from build123d import *

# Parameters (mm, degrees)
SKETCH1_W           = 36.7
SKETCH1_H           = 34.9
SKETCH1_W_2         = 34.7
SKETCH1_H_2         = 32.9
BOSS_EXTRUDE1_DEPTH = 11.2
SKETCH2_W           = 4.9
SKETCH2_H           = 1
CUT_EXTRUDE1_DEPTH  = 1.9
SKETCH4_W           = 36.7
SKETCH4_H           = 34.9
BOSS_EXTRUDE3_DEPTH = 2.5
SKETCH5_W           = 14
SKETCH5_H           = 14
CUT_EXTRUDE2_DEPTH  = 14.7
SKETCH6_W           = 16
SKETCH6_H           = 16
SKETCH6_W_2         = 14
SKETCH6_H_2         = 14
BOSS_EXTRUDE4_DEPTH = 6


with BuildPart() as part:
    # Sketch1 → Boss-Extrude1 (new body)
    with BuildSketch(Plane.XY):
        with Locations((18.35, 17.45)):
            Rectangle(SKETCH1_W, SKETCH1_H)
        with Locations((18.35, 17.45)):
            Rectangle(SKETCH1_W_2, SKETCH1_H_2, mode=Mode.SUBTRACT)
    extrude(amount=BOSS_EXTRUDE1_DEPTH)

    # Sketch2 → Cut-Extrude1 (cut)
    with BuildSketch(Plane(origin=(0, 0, 0), x_dir=(-1, 0, 0), z_dir=(0, 0, -1))):
        with Locations((-28.25, 0.5)):
            Rectangle(SKETCH2_W, SKETCH2_H)
    extrude(amount=-CUT_EXTRUDE1_DEPTH, mode=Mode.SUBTRACT)

    # Sketch4 → Boss-Extrude3 (add)
    with BuildSketch(Plane.XY.offset(11.2)):
        with Locations((18.35, 17.45)):
            Rectangle(SKETCH4_W, SKETCH4_H)
    extrude(amount=BOSS_EXTRUDE3_DEPTH)

    # Sketch5 → Cut-Extrude2 (cut, through all)
    with BuildSketch(Plane.XY.offset(13.7)):
        with Locations((18.3, 18.3)):
            Rectangle(SKETCH5_W, SKETCH5_H)
    extrude(amount=-CUT_EXTRUDE2_DEPTH, mode=Mode.SUBTRACT)

    # Sketch6 → Boss-Extrude4 (add)
    with BuildSketch(Plane(origin=(0, 0, 11.2), x_dir=(-1, 0, 0), z_dir=(0, 0, -1))):
        with Locations((-18.3, 18.3)):
            Rectangle(SKETCH6_W, SKETCH6_H)
        with Locations((-18.3, 18.3)):
            Rectangle(SKETCH6_W_2, SKETCH6_H_2, mode=Mode.SUBTRACT)
    extrude(amount=BOSS_EXTRUDE4_DEPTH)


solid = part.part
Can you work these out from the model? Positions are in its coordinate system, mm. A direction names the side the tool comes from. Give positions to 0.01 mm unless a question says otherwise; leave off trailing zeros. Loops run counter-clockwise (first coordinate to the right, second up) from the corner with the lowest first, then second, coordinate; pieces in that order, holes last. Notation, with made-up numbers: (41, 66.25) -> (48, 66.25) arc R22 ccw to (48, 105.25) -> close; hole circle Ø7 at (-40, 6). An arc over 180 degrees is marked (long way). Use one line per item in the form item = value.
1) We'd pull the mould along Y, two halves only. Please class faces 1 (the face through (18, 34.9, 7)), 2 (the face through (30.7, 0.5, 0.9)), 3 (the face through (18, 1, 6)): released by +Y, released by -Y, zero draft, split by the parting line, or undercut.
Answers:
face_1 = released by +Y
face_2 = zero draft
face_3 = undercut
2) If we section it at D-D (z = 12.5): Please give me the cut outline in (x, y), plus the area to 3 significant figures.
Answers:
outline = (0, 0) -> (36.7, 0) -> (36.7, 34.9) -> (0, 34.9) -> close; hole (11.3, 11.3) -> (25.3, 11.3) -> (25.3, 25.3) -> (11.3, 25.3) -> close
area = 1,080 mm²
3) I need wall thicknesses on line 1 along Y through (x, z) = (15, 10.25); line 2 along Y through (x, z) = (4.5, 8.5); line 3 along X through (y, z) = (22, 13). Which ranges of each line are inside material? Lowest first, please.
Answers:
line_1 = 0 to 1, 10.3 to 11.3, 25.3 to 26.3, 33.9 to 34.9
line_2 = 0 to 1, 33.9 to 34.9
line_3 = 0 to 11.3, 25.3 to 36.7
4) If we section it at C-C (y = 12): Please give me the cut outline in (x, z).
Answers:
outline = (0, 0) -> (1, 0) -> (1, 11.2) -> (10.3, 11.2) -> (10.3, 5.2) -> (11.3, 5.2) -> (11.3, 13.7) -> (0, 13.7) -> close; (25.3, 5.2) -> (26.3, 5.2) -> (26.3, 11.2) -> (35.7, 11.2) -> (35.7, 0) -> (36.7, 0) -> (36.7, 13.7) -> (25.3, 13.7) -> close
5) If we section it at B-B (x = 22): Please give me the cut outline in (y, z).
Answers:
outline = (0, 0) -> (1, 0) -> (1, 11.2) -> (10.3, 11.2) -> (10.3, 5.2) -> (11.3, 5.2) -> (11.3, 13.7) -> (0, 13.7) -> close; (25.3, 5.2) -> (26.3, 5.2) -> (26.3, 11.2) -> (33.9, 11.2) -> (33.9, 0) -> (34.9, 0) -> (34.9, 13.7) -> (25.3, 13.7) -> close
6) If we section it at A-A (z = 8.75): Please give me the cut outline in (x, y), plus the area to 3 significant figures.
Answers:
outline = (0, 0) -> (36.7, 0) -> (36.7, 34.9) -> (0, 34.9) -> close; (10.3, 10.3) -> (26.3, 10.3) -> (26.3, 26.3) -> (10.3, 26.3) -> close; hole (1, 1) -> (35.7, 1) -> (35.7, 33.9) -> (1, 33.9) -> close; hole (11.3, 11.3) -> (25.3, 11.3) -> (25.3, 25.3) -> (11.3, 25.3) -> close
area = 199 mm²
7) Will these pins go through, and if not, where does the flat tip stop? pin 1 (0.8 mm diameter, centred on x = 28.5, y = 0.5, fed in from -Z); pin 2 (3.5 mm diameter, centred on y = 12, z = 6, fed in from -X); pin 3 (1.5 mm diameter, centred on x = 17.5, y = 6.5, fed in from -Z); pin 4 (13 mm diameter, centred on x = 21.5, y = 14.5, fed in from -Z).
Answers:
pin_1 = 1.9
pin_2 = 0
pin_3 = 11.2
pin_4 = 5.2
8) For faces 4 (the face through (18, 10.3, 8)), 5 (the face through (18, 10, 13.7)), 6 (the face through (11.3, 18, 10)), 7 (the face through (0, 17, 7)), 8 (the face through (25.8, 0.5, 0.9)), which set-ups out of +Z, -Z, +X, -X, +Y, -Y let a thin tool reach every point of the face, with its end or its side?
Answers:
face_4 = -Z
face_5 = +Z, +X, -X, +Y, -Y
face_6 = +Z, -Z
face_7 = +Z, -Z, -X, +Y, -Y
face_8 = -Z, -Y
